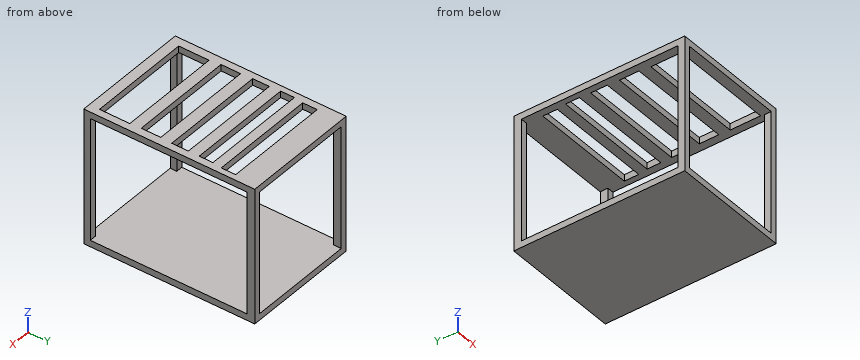
```python
from build123d import *

# Parameters (mm, degrees)
F0_W     = 47.487952
F0_H     = 53.819674
F0_W_2   = 42.307448
F0_H_2   = 48.639174
F1_DEPTH = 68.072
F2_W     = 62.453845
F2_H     = 48.639174
F3_DEPTH = 68.072
F4_W     = 41.156224
F4_H     = 12.087841
F4_W_2   = 41.44403
F4_H_2   = 7.770758
F4_W_3   = 42.01964
F4_H_3   = 6.619532
F4_W_4   = 42.307448
F4_H_4   = 5.468311
F4_W_5   = 42.307446
F4_H_5   = 5.756115
F5_DEPTH = 25.4


with BuildPart() as f1:
    # F0 (on Front) → F1 (new body)
    with BuildSketch(Plane.XZ):
        Rectangle(F0_W, F0_H)
        Rectangle(F0_W_2, F0_H_2, mode=Mode.SUBTRACT)
    extrude(amount=F1_DEPTH)

    # F2 (on face) → F3 (cut)
    with BuildSketch(Plane.YZ.offset(23.743976)):
        with Locations((-34.248885, 0)):
            Rectangle(F2_W, F2_H)
    extrude(amount=-F3_DEPTH, mode=Mode.SUBTRACT)

    # F4 (on face) → F5 (cut)
    with BuildSketch(Plane.XY.offset(26.909837)):
        with Locations((0.273644, -58.007023)):
            Rectangle(F4_W, F4_H)
        with Locations((-0.158064, -43.760637)):
            Rectangle(F4_W_2, F4_H_2)
        with Locations((-0.158064, -31.960601)):
            Rectangle(F4_W_3, F4_H_3)
        with Locations((-0.301968, -21.599593)):
            Rectangle(F4_W_4, F4_H_4)
        with Locations((0.273644, -12.245907)):
            Rectangle(F4_W_5, F4_H_5)
    extrude(amount=-F5_DEPTH, mode=Mode.SUBTRACT)


solid = f1.part
```
Verification items for the finished model (mm, model axes). Give positions to 0.01 mm unless a question says otherwise; leave off trailing zeros. Order: outer loops, then holes, each group sorted by start corner. A loop starts at its lowest first (then second) coordinate and runs counter-clockwise, first axis right, second up. Notation, with made-up numbers: (-25.75, 85) - (19.25, 85) arc R16 cw to (19.25, 111) - close; hole circle Ø8 at (52.5, 68.5). An arc over 180 degrees is marked (long way). Answer as CSV lines item,"result". Start each with the question number.
Item 1: Section check B-B, the plane x = -4.5. Record the boundary of the cut face in (y, z), plus the area to 3 significant figures.
Item 2: Gauge pin test, flat ends, axial feed: pin 1 (3 mm diameter, centred on x = -8, z = 25.5, fed in from +Y); pin 2 (1 mm diameter, centred on x = -1.5, y = -46, fed in from +Z). Record the tip position at first contact, or that the pin passes through.
Item 3: Material ranges on L1, parallel to Z at x = 10, y = -5; L2, parallel to Z at x = -11.5, y = -30.5, recorded low to high.
Item 4: Section check A-A, the plane y = -12. Record the boundary of the cut face in (x, z), plus the area to 3 significant figures.
Item 5: Section check D-D, the plane y = -39. Record the boundary of the cut face in (x, z), plus the area to 3 significant figures.
Item 6: Section check C-C, the plane z = -4. Record the boundary of the cut face in (x, y).
Filled in:
1,outline,"(-68.07, -26.91) - (0, -26.91) - (0, -24.32) - (-68.07, -24.32) - close; (-68.07, 24.32) - (-64.05, 24.32) - (-64.05, 26.91) - (-68.07, 26.91) - close; (-51.96, 24.32) - (-47.65, 24.32) - (-47.65, 26.91) - (-51.96, 26.91) - close; (-39.88, 24.32) - (-35.27, 24.32) - (-35.27, 26.91) - (-39.88, 26.91) - close; (-28.65, 24.32) - (-24.33, 24.32) - (-24.33, 26.91) - (-28.65, 26.91) - close; (-18.87, 24.32) - (-15.12, 24.32) - (-15.12, 26.91) - (-18.87, 26.91) - close; (-9.37, 24.32) - (0, 24.32) - (0, 26.91) - (-9.37, 26.91) - close"
1,area,"255 mm^2"
2,pin 1,"y = 0"
2,pin 2,"z = -24.32"
3,L1,"-26.91 to -24.32, 24.32 to 26.91"
3,L2,"-26.91 to -24.32"
4,outline,"(-23.74, -26.91) - (23.74, -26.91) - (23.74, -24.32) - (-23.74, -24.32) - close; (-23.74, 24.32) - (-20.88, 24.32) - (-20.88, 26.91) - (-23.74, 26.91) - close; (21.43, 24.32) - (23.74, 24.32) - (23.74, 26.91) - (21.43, 26.91) - close"
4,area,"136 mm^2"
5,outline,"(-23.74, -26.91) - (23.74, -26.91) - (23.74, -24.32) - (-23.74, -24.32) - close; (-23.74, 24.32) - (23.74, 24.32) - (23.74, 26.91) - (-23.74, 26.91) - close"
5,area,"246 mm^2"
6,outline,"(-23.74, -68.07) - (-21.15, -68.07) - (-21.15, -65.48) - (-23.74, -65.48) - close; (-23.74, -3.02) - (-21.15, -3.02) - (-21.15, 0) - (-23.74, 0) - close; (21.15, -68.07) - (23.74, -68.07) - (23.74, -65.48) - (21.15, -65.48) - close; (21.15, -3.02) - (23.74, -3.02) - (23.74, 0) - (21.15, 0) - close"
